from build123d import *

# Parameters (mm, degrees)
F1_DEPTH       = 25.4
F3_D           = 7.874
F3_CBORE_D     = 12.7
F3_CBORE_DEPTH = 6.096
F5_DEPTH       = 134.531275
F7_DEPTH       = 118.529275


with BuildPart() as f1:
    # F0 (on Front) → F1 (new body, symmetric)
    with BuildSketch(Plane.XZ):
        Polygon((-91.112512, 12.7), (-91.112512, 0), (-5.260512, 0), (40.590758, -45.85127), (49.571014, -36.871014), (58.55127, -27.890758), (20.474984, 10.185528), (11.494728, 1.205272), (0, 12.7), align=None)
    extrude(amount=F1_DEPTH, both=True)

    # F3 (through all)
    with Locations(Plane(origin=(0, 0, 0), x_dir=(1, 0, 0), z_dir=(0, 0, -1))):
        with Locations((-75.364512, 12.7), (-75.364512, -12.7), (-21.516512, -12.7), (-21.516512, 12.7)):
            CounterBoreHole(F3_D / 2, F3_CBORE_D / 2, F3_CBORE_DEPTH)

    # F4 (on face) → F5 (cut, through all)
    with BuildSketch(Plane(origin=(43.221014, 0, -43.221014), x_dir=(0, 1, 0), z_dir=(0.707107, 0, -0.707107))):
        Polygon((9.652, 21.680256), (-9.652, 21.680256), (-9.652, 15.584256), (-15.748, 15.584256), (-15.748, 8.980256), (15.748, 8.980256), (15.748, 15.584256), (9.652, 15.584256), align=None)
    extrude(amount=-F5_DEPTH, mode=Mode.SUBTRACT)

    # F6 (on face) → F7 (intersect, through all)
    with BuildSketch(Plane(origin=(15.330256, 0, 15.330256), x_dir=(0, 1, 0), z_dir=(0.707107, 0, 0.707107))):
        with BuildLine():
            ThreePointArc((-53.848, -7.275744), (0, -61.123744), (53.848, -7.275744))
            Line((53.848, -7.275744), (-53.848, -7.275744))
        make_face()
        Polygon((-53.848, -7.275744), (53.848, -7.275744), (31.523697, 119.548529), (-64.190522, 119.548529), align=None)
    extrude(amount=-F7_DEPTH, mode=Mode.INTERSECT)


solid = f1.part
Work out the finished part from the listing and answer in its coordinate system (mm). A direction names the side the tool comes from. Round coordinates to 2 decimals unless told otherwise and drop trailing zeros. Write each loop counter-clockwise with the first axis right and the second up, starting at its lowest first coordinate (ties: lowest second). Pieces come first, ordered by that corner, then holes.
1) A cutting plane is placed at D-D (y = 3). Give the vertices of the cut face in (x, z).
2) A cutting plane is placed at A-A (y = -12.7). Give the vertices of the cut face in (x, z) (3 decimals), plus the area to 3 significant figures.
3) The mould has two halves that part along Y. Classify faces 1 (the cylindrical face through (-80.045, -16.992, 3.005)), 2 (the flat face through (39.47, 17.42, -8.81)), 3 (the cylindrical face through (-81.71, 12.42, 3.01)), 4 (the flat face through (-3, 25.4, -2)): pulls with the +Y half, pulls with the -Y half, needs draft (parallel to the pull), parting line crosses it, or undercut.
4) A cutting plane is placed at B-B (z = -3). Give the vertices of the cut face in (x, y).
5) Straight lines are drawn through the part: line 1 (Z direction, x = -62, y = 13.5); line 2 (Y direction, x = 39, z = -23.5); line 3 (X direction, y = -12, z = 2). For each, find the intervals that lie inside material, in ascending order.
6) A tool of negligible diameter and unlimited length cuts with its end or side. For faces 5 (the flat face through (-49, 0, 0)), 6 (the flat face through (37, 9.652, -11)), 7 (the flat face through (32, 15.748, -15)), 8 (the flat face through (17.05, 19.17, 6.76)), from which of +Z, -Z, +X, -X, +Y, -Y can it reach the whole face along a straight path? Write none if from no direction.
7) A cutting plane is placed at C-C (x = -60.5). Give the vertices of the cut face in (y, z), plus the area to 3 significant figures.
8) Given pin 1 Ø12 at (y, z) = (2, -29.5) entering from -X; pin 2 Ø1.5 at (x, y) = (40.5, -8) entering from -Z; pin 3 Ø6.5 at (x, y) = (-22, -10) entering from -Z; pin 4 Ø7 at (x, y) = (-21.52, 12.7) entering from +Z, each flat-ended and moving along its own axis, determine where each tip first touches the part or whether it passes through.
Completed:
1. outline: (-91.11, 0) - (-5.26, 0) - (40.53, -45.79) - (49.51, -36.81) - (0, 12.7) - (-91.11, 12.7) - close
2. outline: (-91.113, 0) - (-81.715, 0) - (-81.715, 6.096) - (-79.302, 6.096) - (-79.302, 12.7) - (-91.113, 12.7) - close; (-71.428, 6.096) - (-69.015, 6.096) - (-69.015, 0) - (-27.867, 0) - (-27.867, 6.096) - (-25.454, 6.096) - (-25.454, 12.7) - (-71.428, 12.7) - close; (-17.58, 6.096) - (-15.167, 6.096) - (-15.167, 0) - (-5.261, 0) - (39.517, -44.777) - (48.497, -35.797) - (0, 12.7) - (-17.58, 12.7) - close; (16.164, 5.875) - (53.167, -31.127) - (57.477, -26.817) - (20.475, 10.186) - close
2. area: 2,020 mm2
3. face 1: undercut
3. face 2: needs draft
3. face 3: undercut
3. face 4: pulls with the +Y half
4. outline: (-2.26, -25.4) - (33.66, -25.4) - (33.66, -9.65) - (25.04, -9.65) - (25.04, -15.75) - (15.7, -15.75) - (15.7, 15.75) - (25.04, 15.75) - (25.04, 9.65) - (33.66, 9.65) - (33.66, 25.4) - (-2.26, 25.4) - close
5. line 1: z = 0 to 12.7
5. line 2: y = -25.4 to -15.75, 15.75 to 25.4
5. line 3: x = -91.11 to -81.68, -69.05 to -27.83, -15.21 to 10.7, 20.04 to 28.66
6. face 5: -Z, -X, +Y, -Y
6. face 6: +Z, +X
6. face 7: none
6. face 8: +Z, +Y, -Y
7. outline: (-25.4, 0) - (25.4, 0) - (25.4, 12.7) - (-25.4, 12.7) - close
7. area: 645 mm2
8. pin 1: stops at x = 18.24
8. pin 2: stops at z = -45.5
8. pin 3: stops at z = 6.1
8. pin 4: passes through
